```python
from build123d import *

# Parameters (mm, degrees)
SKETCH_1_R          = 26.5
EXTRUDE_1_DEPTH     = 5
SKETCH_2_R          = 26.5
SKETCH_2_R_2        = 25
EXTRUDE_2_DEPTH     = 30
SKETCH_3_R          = 2.1
CUT_EXTRUDE_1_DEPTH = 10
EXTRUDE_3_DEPTH     = 2


with BuildPart() as part:
    # 草图1 → 凸台-拉伸1 (new body)
    with BuildSketch(Plane(origin=(0, 0, 0), x_dir=(1, 0, 0), z_dir=(0, 1, 0))):
        with Locations(Location((0, 0, 0), (0, 0, 270))):
            Circle(SKETCH_1_R)
    extrude(amount=EXTRUDE_1_DEPTH)

    # 草图2 → 凸台-拉伸2 (add)
    with BuildSketch(Plane(origin=(0, 5, 0), x_dir=(1, 0, 0), z_dir=(0, 1, 0))):
        with Locations(Location((0, 0, 0), (0, 0, 270))):
            Circle(SKETCH_2_R)
        with Locations(Location((0, 0, 0), (0, 0, 270))):
            Circle(SKETCH_2_R_2, mode=Mode.SUBTRACT)
    extrude(amount=EXTRUDE_2_DEPTH)

    # 草图3 → 切除-拉伸1 (cut)
    with BuildSketch(Plane.XZ):
        with Locations(Location((0, 0, 0), (0, 0, 270))):
            Circle(SKETCH_3_R)
    extrude(amount=-CUT_EXTRUDE_1_DEPTH, mode=Mode.SUBTRACT)

    # 草图4 → 凸台-拉伸3 (add)
    with BuildSketch(Plane(origin=(0, 5, 0), x_dir=(1, 0, 0), z_dir=(0, 1, 0))):
        with BuildLine():
            ThreePointArc((-13.829204077, -2.180163894), (-13.314791228, 4.326237921), (-9.906592932, 9.892391848))
            Line((-9.906592932, 9.892391848), (-11.421352179, 11.97727909))
            ThreePointArc((-11.421352179, 11.97727909), (-15.739985345, 5.114231257), (-16.280136023, -2.976519958))
            Line((-16.280136023, -2.976519958), (-13.829204077, -2.180163894))
        make_face()
        with BuildLine():
            ThreePointArc((-6.346918157, 12.478646958), (0, 14), (6.346918157, 12.478646958))
            Line((6.346918157, 12.478646958), (7.861677404, 14.5635342))
            ThreePointArc((7.861677404, 14.5635342), (0, 16.55), (-7.861677404, 14.5635342))
            Line((-7.861677404, 14.5635342), (-6.346918157, 12.478646958))
        make_face()
        with BuildLine():
            ThreePointArc((14, 0), (13.957235705, -1.093421906), (13.829204077, -2.180163894))
            Line((13.829204077, -2.180163894), (16.280136023, -2.976519958))
            ThreePointArc((16.280136023, -2.976519958), (16.48239593, -1.494364215), (16.55, 0))
            ThreePointArc((16.55, 0), (15.213906115, 6.514565275), (11.421352179, 11.97727909))
            Line((11.421352179, 11.97727909), (9.906592932, 9.892391848))
            ThreePointArc((9.906592932, 9.892391848), (12.936234016, 5.352929056), (14, 0))
        make_face()
        with BuildLine():
            ThreePointArc((12.469529301, -6.364812566), (8.228993532, -11.326237921), (2.2, -13.826062346))
            Line((2.2, -13.826062346), (2.2, -16.403124702))
            ThreePointArc((2.2, -16.403124702), (9.727845925, -13.389231257), (14.920461248, -7.16116863))
            Line((14.920461248, -7.16116863), (12.469529301, -6.364812566))
        make_face()
        with BuildLine():
            Line((-2.2, -16.403124702), (-2.2, -13.826062346))
            ThreePointArc((-2.2, -13.826062346), (-8.228993532, -11.326237921), (-12.469529301, -6.364812566))
            Line((-12.469529301, -6.364812566), (-14.920461248, -7.16116863))
            ThreePointArc((-14.920461248, -7.16116863), (-9.727845925, -13.389231257), (-2.2, -16.403124702))
        make_face()
    extrude(amount=EXTRUDE_3_DEPTH)


solid = part.part
```
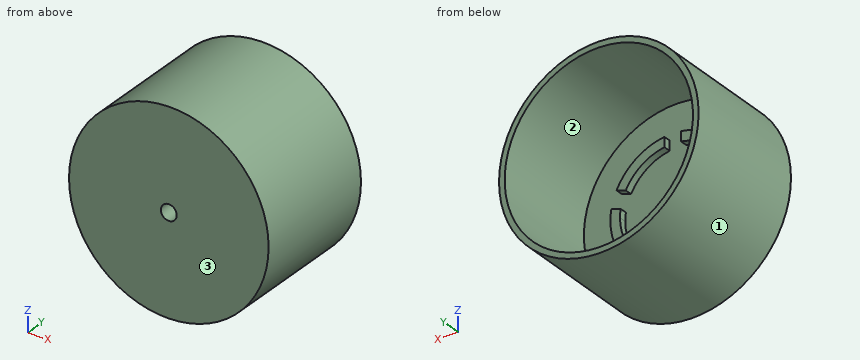
Check sheet for the modelled part. Datum: model origin and axes. Units: mm. Face numbers are marked on the shaded views. Round coordinates to 2 decimals unless told otherwise and drop trailing zeros. Order: outer loops, then holes, each group sorted by start corner. A loop starts at its lowest first (then second) coordinate and runs counter-clockwise, first axis right, second up. Notation, with made-up numbers: (-32.75, -11) -> (-15.75, -11) arc R24 cw to (-15.75, 10) -> close; hole circle Ø8 at (-4, -9.75). An arc over 180 degrees is marked (long way). One line per item, written item: value. Start each with the question number.
Q1. Cross-section at B-B (y = 28). Record the boundary of the cut face in (x, z).
Q2. Mould release check, pull along X, two halves, no side actions. Record for the marked faces 1, 2 and 3: pulls with the +X half, pulls with the -X half, needs draft (parallel to the pull), parting line crosses it, or undercut.
Q3. Gauge pin test, flat ends, axial feed: pin 1 Ø1.5 at (y, z) = (20.5, -11.5) entering from -X; pin 2 Ø6 at (y, z) = (10.5, 20.5) entering from +X; pin 3 Ø7.5 at (x, z) = (13, -7) entering from +Y. Record the tip position at first contact, or that the pin passes through.
Q4. Thickness scan on line 1 (X direction, y = 1.75, z = 0); line 2 (Y direction, x = -7.5, z = -1); line 3 (X direction, y = 24.75, z = 0). Record the ranges inside material, lowest first.
Q5. Cross-section at C-C (z = 20.5). Record the boundary of the cut face in (x, y), and give its area (3 significant figures).
Q6. Cross-section at A-A (x = 0). Record the boundary of the cut face in (y, z), and give its area (3 significant figures).
Q7. Cross-section at D-D (x = 9). Record the boundary of the cut face in (y, z).
Completed:
1. outline: circle Ø53 at (0, 0); hole circle Ø50 at (0, 0)
2. face 1: parting line crosses it
2. face 2: undercut
2. face 3: needs draft
3. pin 1: stops at x = -24.22
3. pin 2: stops at x = 19.9
3. pin 3: stops at y = 7
4. line 1: x = -26.5 to -2.1, 2.1 to 26.5
4. line 2: y = 0 to 5
4. line 3: x = -26.5 to -25, 25 to 26.5
5. outline: (-16.79, 0) -> (16.79, 0) -> (16.79, 35) -> (14.31, 35) -> (14.31, 5) -> (-14.31, 5) -> (-14.31, 35) -> (-16.79, 35) -> close
5. area: 317 mm²
6. outline: (0, -26.5) -> (35, -26.5) -> (35, -25) -> (5, -25) -> (5, -16.55) -> (7, -16.55) -> (7, -14) -> (5, -14) -> (5, -2.1) -> (0, -2.1) -> close; (0, 2.1) -> (5, 2.1) -> (5, 25) -> (35, 25) -> (35, 26.5) -> (0, 26.5) -> close
6. area: 339 mm²
7. outline: (0, -24.92) -> (35, -24.92) -> (35, -23.32) -> (5, -23.32) -> (5, 10.72) -> (7, 10.72) -> (7, 13.89) -> (5, 13.89) -> (5, 23.32) -> (35, 23.32) -> (35, 24.92) -> (0, 24.92) -> close
